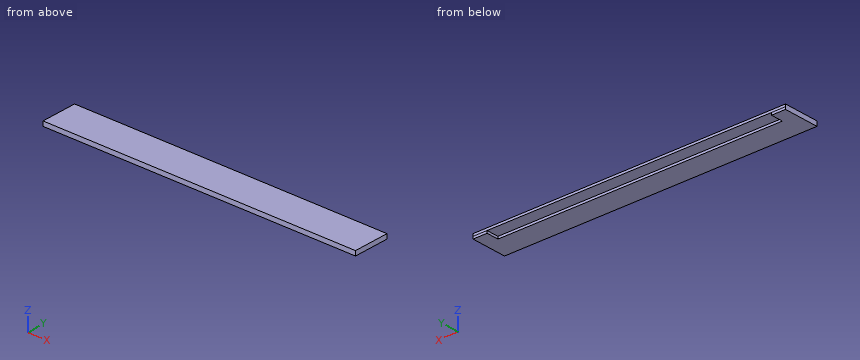
Autodesk Inventor part; units mm, degrees
ref_plane "YZ Plane" through (0, 0, 0) normal (1, 0, 0) x (0, 1, 0)
ref_plane "XZ Plane" through (0, 0, 0) normal (0, 1, 0) x (-1, 0, 0)
ref_plane "XY Plane" through (0, 0, 0) normal (0, 0, 1) x (1, 0, 0)
sketch "Sketch1" plane through (0, 0, 0) normal (1, 0, 0) x (0, 1, 0)
  line L0 (0, 0) -> (155.1, 0)
  line L1 (155.1, 0) -> (155.1, -10)
  line L2 (0, -20) -> (0, 0)
  line L3 (155.1, -10) -> (101.6, -10)
  line L4 (101.6, -10) -> (101.6, -20)
  line L5 (101.6, -20) -> (0, -20)
  dimension "d3" = 53.5
  dimension "d4" = 155.1
  dimension "d5" = 10
  dimension "d6" = 10
  dimension "d7" = 20
  dimension "d18" = 101.6
extrude "Extrusion1" add sketch "Sketch1" along normal blind 1350.7974
sketch "Sketch3" plane through (0, 101.6, -10) normal (0, 1, 0) x (1, 0, 0)
  line L0 (1350.7974, -10) -> (1350.7974, 10)
  line L1 (1350.7974, 10) -> (1289.9898, 10)
  line L2 (1289.9898, 10) -> (1289.9898, 0)
  line L3 (0, 0) -> (1350.7974, 0)
  line L4 (0, 10) -> (0, -10)
  line L5 (0, 10) -> (60.8076, 10)
  line L6 (60.8076, 10) -> (60.8076, 0)
  dimension "d19" = 60.8076
  dimension "d20" = 60.8076
extrude "Extrusion2" add sketch "Sketch3" along normal blind 53.4924 contours L3 L2 L1 L0
sketch "Sketch4" plane through (0, 101.6, -20) normal (0, 1, 0) x (1, 0, 0)
  line L0 (1350.7974, -10) -> (1350.7974, 10)
  line L1 (1350.7974, 10) -> (1289.9898, 10)
  line L2 (1289.9898, 10) -> (1289.9898, 0)
  line L3 (0, 0) -> (1350.7974, 0)
  line L4 (0, 10) -> (60.8076, 10)
  line L5 (60.8076, 10) -> (60.8076, 0)
  line L6 (0, 10) -> (0, 0)
  line L7 (0, -20) -> (0, -10)
  line L8 (0, 0) -> (0, -20)
  line L9 (60.8076, 0) -> (60.8076, -10)
  line L10 (0, -10) -> (1350.7974, -10)
  line L11 (0, -10) -> (60.8076, -10)
  line L12 (0, -10) -> (0, 0)
  dimension "d23" = 60.8076
  dimension "d24" = 60.8076
  dimension "d25" = 10
  dimension "d26" = 20
extrude "Extrusion3" add sketch "Sketch4" along normal blind 53.4924 contours L10 L8 L3 L9
properties part number "SkinnySideL" material "Wood (Birch)"
Could you check a few things on this model? Use its own coordinates, in mm. Coordinates: 2 decimals unless noted, no trailing zeros. Order: outer loops, then holes, each group sorted by start corner. A loop starts at its lowest first (then second) coordinate and runs counter-clockwise, first axis right, second up. Notation, with made-up numbers: (-32.5, 32.25) -> (-7.5, 32.25) arc R35 ccw to (-7.5, 68.25) -> close; hole circle Ø8 at (27.25, -15.75). An arc over 180 degrees is marked (long way). One line per item, written item: value. Start each with the question number.
1) I'm going to push flat-ended pins straight in: pin 1 (12 mm diameter, centred on x = 390.5, z = -17, fed in from +Y); pin 2 (11 mm diameter, centred on x = 1327, z = -17, fed in from +Y). Where does each tip first touch, or does it pass through?
2) Imagine slicing it at A-A on z = -16.75. List the corners of the cut face in (x, y) for me, plus the area to 3 significant figures.
3) Imagine slicing it at B-B on y = 128.5. List the corners of the cut face in (x, z) for me.
4) If I drill on L1, parallel to X at y = 130, z = -18; L2, parallel to Y at x = 992, z = -13.5; L3, parallel to Z at x = 1160.5, y = 146.5, over which ranges is the centre line in solid material (lowest first)? Write a range as [from, to].
5) Imagine slicing it at C-C on x = 485.5. List the corners of the cut face in (y, z) for me.
Answer list:
1. pin 1: stops at y = 101.6
1. pin 2: stops at y = 155.09
2. outline: (0, 0) -> (1350.8, 0) -> (1350.8, 155.09) -> (1289.99, 155.09) -> (1289.99, 101.6) -> (60.81, 101.6) -> (60.81, 155.09) -> (0, 155.09) -> close
2. area: 144,000 mm2
3. outline: (0, -20) -> (60.81, -20) -> (60.81, -10) -> (1289.99, -10) -> (1289.99, -20) -> (1350.8, -20) -> (1350.8, 0) -> (0, 0) -> close
4. L1: x = [0, 60.81], [1289.99, 1350.8]
4. L2: y = [0, 101.6]
4. L3: z = [-10, 0]
5. outline: (0, -20) -> (101.6, -20) -> (101.6, -10) -> (155.1, -10) -> (155.1, 0) -> (0, 0) -> close
